from build123d import *

# Parameters (mm, degrees)
SKETCH1_R           = 63.5
BOSS_EXTRUDE1_DEPTH = 76.2
SKETCH2_R           = 57.15
CUT_EXTRUDE1_DEPTH  = 69.85
SKETCH4_R           = 25.4
BOSS_EXTRUDE2_DEPTH = 25.4
SKETCH5_R           = 22.225
CUT_EXTRUDE2_DEPTH  = 2514.6
SKETCH8_R           = 63.5
BOSS_EXTRUDE3_DEPTH = 25.4
SKETCH9_R           = 57.15
CUT_EXTRUDE3_DEPTH  = 50.8
BOSS_EXTRUDE5_DEPTH = 25.4
BOSS_EXTRUDE6_DEPTH = 25.4
SKETCH14_R          = 1.389063
CUT_EXTRUDE4_DEPTH  = 2514.6


with BuildPart() as part:
    # Sketch1 → Boss-Extrude1 (new body)
    with BuildSketch(Plane(origin=(0, 0, 0), x_dir=(1, 0, 0), z_dir=(0, 1, 0))):
        Circle(SKETCH1_R)
    extrude(amount=BOSS_EXTRUDE1_DEPTH)

    # Sketch2 → Cut-Extrude1 (cut)
    with BuildSketch(Plane(origin=(0, 76.2, 0), x_dir=(1, 0, 0), z_dir=(0, 1, 0))):
        Circle(SKETCH2_R)
    extrude(amount=-CUT_EXTRUDE1_DEPTH, mode=Mode.SUBTRACT)

    # Sketch4 → Boss-Extrude2 (add)
    with BuildSketch(Plane.XZ):
        Circle(SKETCH4_R)
    extrude(amount=BOSS_EXTRUDE2_DEPTH)

    # Sketch5 → Cut-Extrude2 (cut)
    with BuildSketch(Plane.XZ.offset(25.4)):
        Circle(SKETCH5_R)
    extrude(amount=-CUT_EXTRUDE2_DEPTH, mode=Mode.SUBTRACT)

    # Sketch8 → Boss-Extrude3 (add)
    with BuildSketch(Plane(origin=(0, 76.2, 0), x_dir=(1, 0, 0), z_dir=(0, 1, 0))):
        Circle(SKETCH8_R)
    extrude(amount=BOSS_EXTRUDE3_DEPTH)

    # Sketch9 → Cut-Extrude3 (cut)
    with BuildSketch(Plane(origin=(0, 101.6, 0), x_dir=(1, 0, 0), z_dir=(0, 1, 0))):
        Circle(SKETCH9_R)
    extrude(amount=-CUT_EXTRUDE3_DEPTH, mode=Mode.SUBTRACT)

    # Sketch11 → Boss-Extrude5 (add)
    with BuildSketch(Plane(origin=(0, 101.6, 0), x_dir=(1, 0, 0), z_dir=(0, 1, 0))):
        with BuildLine():
            Line((-61.976, 13.828428), (-55.372, 14.144402))
            ThreePointArc((-55.372, 14.144402), (-57.15, 0), (-55.372, -14.144402))
            Line((-55.372, -14.144402), (-61.976, -13.828428))
            ThreePointArc((-61.976, -13.828428), (-63.5, 0), (-61.976, 13.828428))
        make_face()
    extrude(amount=BOSS_EXTRUDE5_DEPTH)

    # Sketch13 → Boss-Extrude6 (add)
    with BuildSketch(Plane(origin=(0, 101.6, 0), x_dir=(1, 0, 0), z_dir=(0, 1, 0))):
        with BuildLine():
            Line((55.372, 14.144402), (61.976, 13.828428))
            ThreePointArc((61.976, 13.828428), (63.5, 0), (61.976, -13.828428))
            Line((61.976, -13.828428), (55.372, -14.144402))
            ThreePointArc((55.372, -14.144402), (57.15, 0), (55.372, 14.144402))
        make_face()
    extrude(amount=BOSS_EXTRUDE6_DEPTH)

    # Sketch14 → Cut-Extrude4 (cut)
    with BuildSketch(Plane(origin=(101.6, 0, 0), x_dir=(0, 0, -1), z_dir=(1, 0, 0))):
        with Locations((0.081717, 115.219319)):
            Circle(SKETCH14_R)
    extrude(amount=-CUT_EXTRUDE4_DEPTH, mode=Mode.SUBTRACT)


solid = part.part
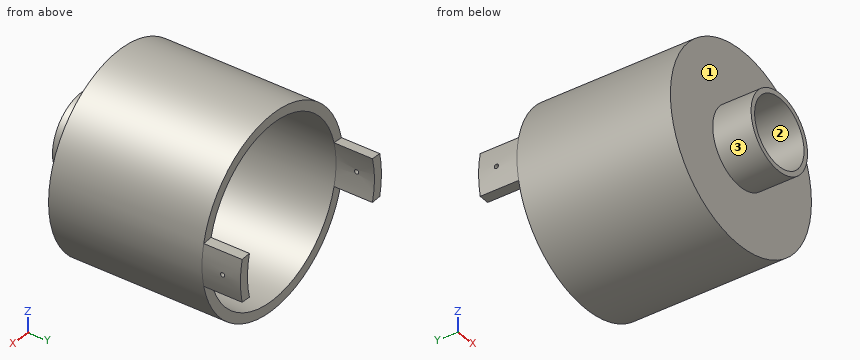
Can you work these out from the model? Positions are in its coordinate system, mm. Face numbers are marked on the shaded views. Coordinates: 2 decimals unless noted, no trailing zeros. Write each loop counter-clockwise with the first axis right and the second up, starting at its lowest first coordinate (ties: lowest second). Pieces come first, ordered by that corner, then holes. Notation, with made-up numbers: (-28, 86) -> (24, 86) arc R16 cw to (24, 113) -> close; hole circle Ø10 at (47, 45). An arc over 180 degrees is marked (long way). Write each question's results on one line, items separated by ' | '. Start each with the question number.
Q1. Imagine slicing it at A-A (y = 108.5). Write out the boundary of the cut face in (x, z).
Q2. We'd pull the mould along Z, two halves only. Please class the marked faces 1, 2 and 3: +Z half, -Z half, draft (parallel to the pull), parting line (faces both ways), or undercut.
Q3. Imagine slicing it at D-D (y = 60.5). Write out the boundary of the cut face in (x, z).
Q4. Imagine slicing it at B-B (x = 0). Write out the boundary of the cut face in (y, z) (3 decimals), then the cut area to 3 significant figures.
Q5. If I drill on probe 1 along X at (y, z) = (59, 0); probe 2 along X at (y, z) = (52, -14); probe 3 along Z at (x, y) = (0, -5.5) (3 decimals), over which ranges is the centre line in solid material (lowest first)?
Q6. I'm going to push flat-ended pins straight in: pin 1 (1 mm diameter, centred on x = -33.5, y = 77, fed in from -Z); pin 2 (4 mm diameter, centred on y = 8, z = 46.5, fed in from +X); pin 3 (5 mm diameter, centred on x = -43, z = 45.5, fed in from +Y). Where does each tip first touch, or does it pass through?
Q7. Imagine slicing it at C-C (z = 3.5). Write out the boundary of the cut face in (x, y).
Taken from the geometry:
1) outline: (-61.98, -13.83) -> (-55.37, -14.14) arc R57.15 cw to (-55.37, 14.14) -> (-61.98, 13.83) arc R63.5 ccw to start; (55.37, -14.14) -> (61.98, -13.83) arc R63.5 ccw to (61.98, 13.83) -> (55.37, 14.14) arc R57.15 cw to start
2) face 1: draft | face 2: undercut | face 3: parting line
3) outline: circle Ø127 at (0, 0); hole circle Ø114.3 at (0, 0)
4) outline: (-25.4, -25.4) -> (0, -25.4) -> (0, -63.5) -> (101.6, -63.5) -> (101.6, -57.15) -> (6.35, -57.15) -> (6.35, -22.225) -> (-25.4, -22.225) -> close; (-25.4, 22.225) -> (6.35, 22.225) -> (6.35, 57.15) -> (101.6, 57.15) -> (101.6, 63.5) -> (0, 63.5) -> (0, 25.4) -> (-25.4, 25.4) -> close | area: 1,900 mm^2
5) probe 1: x = -63.5 to -57.15, 57.15 to 63.5 | probe 2: x = -61.94 to -55.41, 55.41 to 61.94 | probe 3: z = -25.4 to -22.225, 22.225 to 25.4
6) pin 1: stops at z = -54.25 | pin 2: stops at x = 45.3 | pin 3: stops at y = 101.6
7) outline: (-63.4, 0) -> (-25.16, 0) -> (-25.16, -25.4) -> (-21.95, -25.4) -> (-21.95, 6.35) -> (-57.04, 6.35) -> (-57.04, 127) -> (-63.4, 127) -> close; (21.95, -25.4) -> (25.16, -25.4) -> (25.16, 0) -> (63.4, 0) -> (63.4, 127) -> (57.04, 127) -> (57.04, 6.35) -> (21.95, 6.35) -> close
